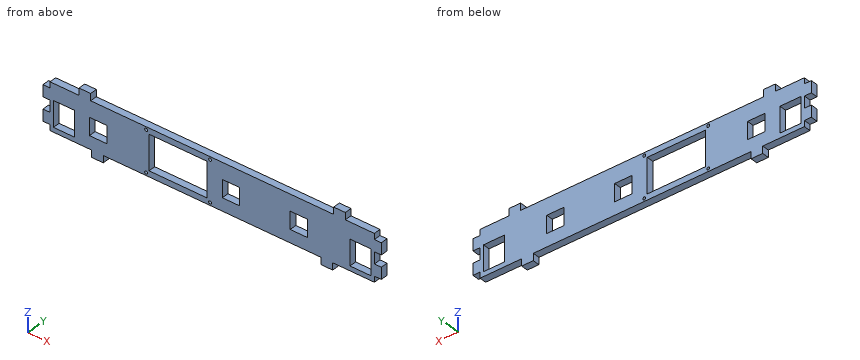
from build123d import *

# Parameters (mm, degrees)
F0_R     = 1.25
F0_W     = 18
F0_H     = 22
F0_W_2   = 15
F0_H_2   = 15
F0_W_3   = 50
F0_H_3   = 30
F1_DEPTH = 6


with BuildPart() as f1:
    # F0 (on Front) → F1 (new body)
    with BuildSketch(Plane.XZ):
        Polygon((-139.5, -13.727578), (-139.5, -18.727578), (-103.67224, -18.727578), (-103.67224, -24.727578), (-93.67224, -24.727578), (-93.67224, -18.727578), (0, -18.727578), (93.67224, -18.727578), (93.67224, -24.727578), (103.67224, -24.727578), (103.67224, -18.727578), (139.5, -18.727578), (139.5, -13.727578), (145.5, -13.727578), (145.5, -3.727578), (139.5, -3.727578), (139.5, 6.272422), (145.5, 6.272422), (145.5, 16.272422), (139.499999, 16.272422), (139.49919, 21.272422), (114.49919, 21.272422), (114.49919, 27.272422), (104.49919, 27.272422), (104.49919, 21.272422), (0, 21.272422), (-104.49919, 21.272422), (-104.49919, 27.272422), (-114.49919, 27.272422), (-114.49919, 21.272422), (-139.49919, 21.272422), (-139.499999, 16.272422), (-145.5, 16.272422), (-145.5, 6.272422), (-139.5, 6.272422), (-139.5, -3.727578), (-145.5, -3.727578), (-145.5, -13.727578), align=None)
        with Locations((-56.8, -16.227578)):
            Circle(F0_R, mode=Mode.SUBTRACT)
        with Locations((-1.8, -16.227578)):
            Circle(F0_R, mode=Mode.SUBTRACT)
        with Locations((-127.5, -3.727578)):
            Rectangle(F0_W, F0_H, mode=Mode.SUBTRACT)
        with Locations((-98.1, -0.227578)):
            Rectangle(F0_W_2, F0_H_2, mode=Mode.SUBTRACT)
        with Locations((16.2, -0.227578)):
            Rectangle(F0_W_2, F0_H_2, mode=Mode.SUBTRACT)
        with Locations((74.6, -0.227578)):
            Rectangle(F0_W_2, F0_H_2, mode=Mode.SUBTRACT)
        with Locations((127.5, -3.727578)):
            Rectangle(F0_W, F0_H, mode=Mode.SUBTRACT)
        with Locations((-29.3, 1.272422)):
            Rectangle(F0_W_3, F0_H_3, mode=Mode.SUBTRACT)
        with Locations((-56.8, 18.772422)):
            Circle(F0_R, mode=Mode.SUBTRACT)
        with Locations((-1.8, 18.772422)):
            Circle(F0_R, mode=Mode.SUBTRACT)
    extrude(amount=F1_DEPTH)


solid = f1.part
Can you work these out from the model? Positions are in its coordinate system, mm. Coordinates: 2 decimals unless noted, no trailing zeros. Write each loop counter-clockwise with the first axis right and the second up, starting at its lowest first coordinate (ties: lowest second). Pieces come first, ordered by that corner, then holes. Notation, with made-up numbers: (-35.5, -26.5) - (-15.5, -26.5) arc R25 ccw to (-15.5, -5.5) - close; hole circle Ø4 at (2.25, 85). An arc over 180 degrees is marked (long way). Return JSON: item names as keys, results as strings. Group by question number.
Item 1: If we section it at D-D (x = -72): Write out the boundary of the cut face in (y, z).
Item 2: If we section it at A-A (z = -1): Write out the boundary of the cut face in (x, y).
Item 3: If we section it at B-B (x = 14): Write out the boundary of the cut face in (y, z).
Item 4: Please list where these lines run through material, in increasing order: probe 1 along Z at (x, y) = (-1.8, -3.8); probe 2 along X at (y, z) = (-2.65, -21); probe 3 along Z at (x, y) = (-12.5, -2.15).
Item 5: If we section it at C-C (y = -3.35): Count the separate pieces of the cut face and the enclosed holes in it, then the cut area to 3 significant figures.
Item 6: I'm going to push flat-ended pins straight in: pin 1 Ø1.8 at (y, z) = (-2, 2) entering from -X; pin 2 Ø1.8 at (x, y) = (71, -3.5) entering from +Z; pin 3 Ø5 at (x, z) = (13, -5) entering from -Y; pin 4 Ø1.8 at (y, z) = (-3.5, 25) entering from +X. Where does each tip first touch, or does it pass through?
Return value:
{
 "1": {"outline": "(-6, -18.73) - (0, -18.73) - (0, 21.27) - (-6, 21.27) - close"},
 "2": {"outline": "(-139.5, -6) - (-136.5, -6) - (-136.5, 0) - (-139.5, 0) - close; (-118.5, -6) - (-105.6, -6) - (-105.6, 0) - (-118.5, 0) - close; (-90.6, -6) - (-54.3, -6) - (-54.3, 0) - (-90.6, 0) - close; (-4.3, -6) - (8.7, -6) - (8.7, 0) - (-4.3, 0) - close; (23.7, -6) - (67.1, -6) - (67.1, 0) - (23.7, 0) - close; (82.1, -6) - (118.5, -6) - (118.5, 0) - (82.1, 0) - close; (136.5, -6) - (139.5, -6) - (139.5, 0) - (136.5, 0) - close"},
 "3": {"outline": "(-6, -18.73) - (0, -18.73) - (0, -7.73) - (-6, -7.73) - close; (-6, 7.27) - (0, 7.27) - (0, 21.27) - (-6, 21.27) - close"},
 "4": {"probe 1": "z = -18.73 to -17.48, -14.98 to 17.52, 20.02 to 21.27", "probe 2": "x = -103.67 to -93.67, 93.67 to 103.67", "probe 3": "z = -18.73 to -13.73, 16.27 to 21.27"},
 "5": {"separate pieces": "1", "enclosed holes": "10", "area": "8,650 mm^2"},
 "6": {"pin 1": "stops at x = -139.5", "pin 2": "stops at z = 21.27", "pin 3": "passes through", "pin 4": "stops at x = 114.5"}
}
